Geometry check sheet. Reference: drawing and pictorial views, mm from the part's lowest x, y, z. A direction names the side the tool comes from. Give positions to 0.01 mm unless a question says otherwise; leave off trailing zeros. Order: outer loops, then holes, each group sorted by start corner. A loop starts at its lowest first (then second) coordinate and runs counter-clockwise, first axis right, second up. Notation, with made-up numbers: M 47.5,-9.5 L 77.5,-9.5 A11 ccw 77.5,2.5 Z; hole C -10,-0.75 d6. An arc over 180 degrees is marked long. Answer as a JSON object with one key per item and string values. Group by question number.
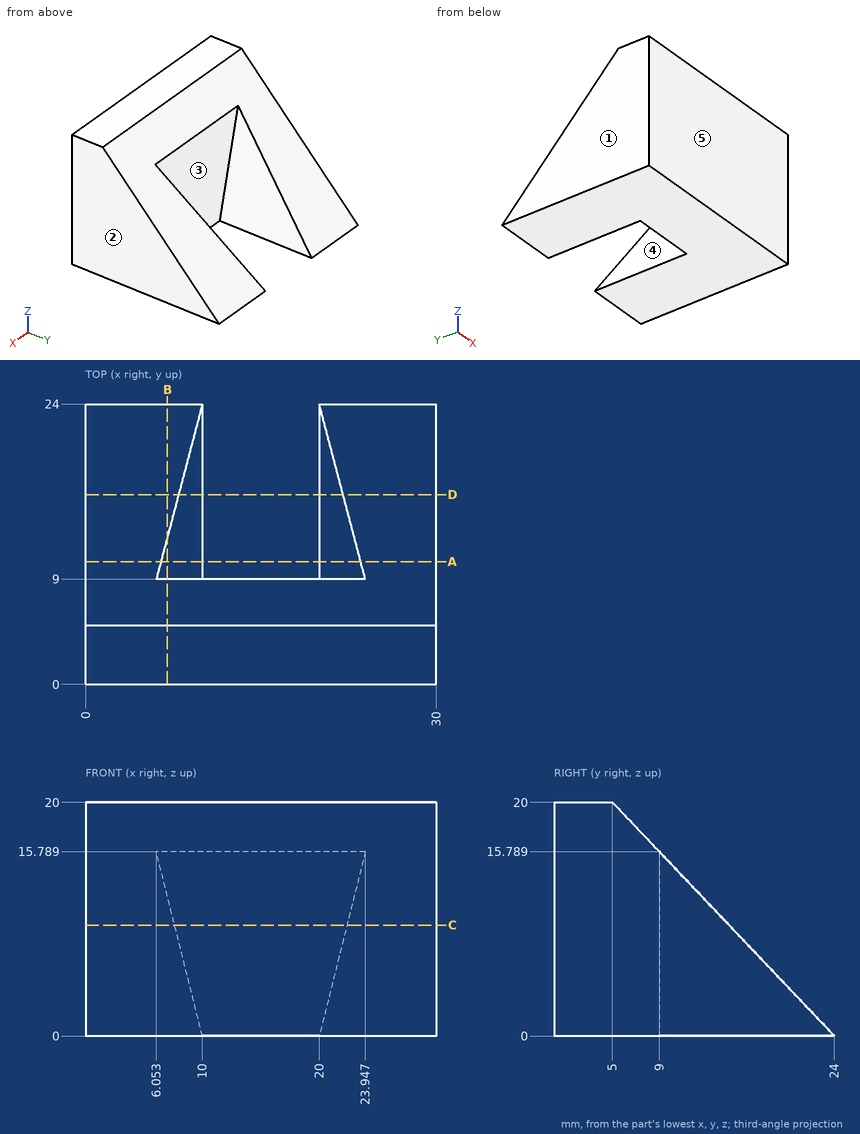
1. Cross-section at A-A (y = 10.5). Record the cut outline in (x, z), and give its area (3 significant figures).
2. Release check for a two-part mould opening along X. For the marked faces 1, 2 and 3 record: released by +X, released by -X, zero draft, split by the parting line, or undercut.
3. Thickness scan on line 1 along X through (y, z) = (15.5, 2.25); line 2 along X through (y, z) = (15.5, 2); line 3 along Y through (x, z) = (15, 8.75). Record the ranges inside material, lowest first. Write a range as [from, to].
4. Cross-section at B-B (x = 7). Record the cut outline in (y, z).
5. Depth check by flat-ended pin: pin 1 (12 mm diameter, centred on x = 6.5, z = 9, fed in from +Y); pin 2 (1.5 mm diameter, centred on x = 6, z = 15.5, fed in from +Y); pin 3 (1.5 mm diameter, centred on x = 24.5, z = 5, fed in from +Y). Enter the tip coordinate at first touch or a pass-through.
6. Cross-section at C-C (z = 9.5). Record the cut outline in (x, y) (1 decimal), and give its area (3 significant figures).
7. Access from +Z, -Z, +X, -X, +Y, -Y to the whole of each face (thin tool, end or side, straight path). Record for the marked faces 4 and 5.
8. Cross-section at D-D (y = 16.25). Record the cut outline in (x, z).
Report:
{
 "1": {"outline": "M 0,0 L 10,0 L 6.45,14.21 L 0,14.21 Z; M 20,0 L 30,0 L 30,14.21 L 23.55,14.21 Z", "area": "234 mm2"},
 "2": {"face 1": "released by -X", "face 2": "released by +X", "face 3": "undercut"},
 "3": {"line 1": "x = [0, 9.44], [20.56, 30]", "line 2": "x = [0, 9.5], [20.5, 30]", "line 3": "y = [0, 9]"},
 "4": {"outline": "M 0,0 L 24,0 L 12.6,12 L 9,12 L 9,15.79 L 5,20 L 0,20 Z"},
 "5": {"pin 1": "stops at y = 21.15", "pin 2": "stops at y = 9.99", "pin 3": "stops at y = 19.96"},
 "6": {"outline": "M 0,0 L 30,0 L 30,15 L 22.4,15 L 22.4,9 L 7.6,9 L 7.6,15 L 0,15 Z", "area": "361 mm2"},
 "7": {"face 4": "+Z, +Y", "face 5": "+Z, -Z, +X, -X, -Y"},
 "8": {"outline": "M 0,0 L 10,0 L 7.96,8.16 L 0,8.16 Z; M 20,0 L 30,0 L 30,8.16 L 22.04,8.16 Z"}
}
